CAD build for the part. Positions are in the model's coordinates, mm. A direction names the side the tool comes from. Coordinates: 2 decimals unless noted, no trailing zeros. Order: outer loops, then holes, each group sorted by start corner. A loop starts at its lowest first (then second) coordinate and runs counter-clockwise, first axis right, second up. Notation, with made-up numbers: M 87.25,64 L 140.25,64 A12 cw 140.25,73 Z; hole C 57.25,-2 d8. An arc over 180 degrees is marked long. Write item = value, one per line. Start each with the question number.
```python
from build123d import *

# Parameters (mm, degrees)
F0_W     = 82
F0_H     = 20
F0_R     = 2.5
F0_R_2   = 3
F1_DEPTH = 10
F2_W     = 57
F2_H     = 2
F3_DEPTH = 10


# Not quite as in the source:
# - a feature names something its author has since deleted; it is built from what else it names


with BuildPart() as f1:
    # F0 (on Top) → F1 (new body)
    with BuildSketch(Plane.XY):
        Rectangle(F0_W, F0_H)
        with Locations((26, -5)):
            Circle(F0_R, mode=Mode.SUBTRACT)
        with Locations((36, -5)):
            Circle(F0_R, mode=Mode.SUBTRACT)
        with Locations((-8, 0)):
            Circle(F0_R_2, mode=Mode.SUBTRACT)
    extrude(amount=F1_DEPTH)

    # F2 (on face) → F3 (cut)
    with BuildSketch(Plane.XY.offset(10)):
        Polygon((-16, 10), (-41, 10), (-41, -2), (-16, -2), (-16, 8), align=None)
        with Locations((12.5, 9)):
            Rectangle(F2_W, F2_H)
    extrude(amount=-F3_DEPTH, mode=Mode.SUBTRACT)


solid = f1.part
```
1. Slice it at D-D (y = -5). Write the cut outline in (x, z).
2. Slice it at A-A (y = 0). Write the cut outline in (x, z).
3. Slice it at B-B (x = -8). Write the cut outline in (y, z), plus the area to 3 significant figures.
4. Slice it at C-C (z = 2.5). Write the cut outline in (x, y).
5. Probe L1, parallel to Y at x = -8, z = 7.75; L2, parallel to Y at x = 36, z = 4.5; L3, parallel to X at y = -4, z = 0.75. List the from-to ranges inside material, lowest first.
6. 3-axis set-ups, long thin cutter, end or side, ignore diameter. For faces 1 (the flat face through (-41, -6, 5)), 2 (the flat face through (-16, 3, 5)): which of +Z, -Z, +X, -X, +Y, -Y reach the whole face in a straight line?
7. Mould opens along Y. For faces 3 (the flat face through (-29, -2, 5)), 4 (the flat face through (-1, -1, 10)), 5 (the cylindrical face through (24.16, -3.31, 4.93)) say: released by +Y, released by -Y, zero draft, split by the parting line, or undercut.
8. Flat gauge pins, fed straight in: pin 1 (5 mm diameter, centred on x = -32.5, z = 4, fed in from +Y); pin 2 (3.5 mm diameter, centred on x = -8, y = 0, fed in from +Z); pin 3 (3 mm diameter, centred on y = 0.5, z = 4.5, fed in from -X). Where does each tip first touch, or does it go through?
Calculated:
q1.outline = M -41,0 L 23.5,0 L 23.5,10 L -41,10 Z; M 28.5,0 L 33.5,0 L 33.5,10 L 28.5,10 Z; M 38.5,0 L 41,0 L 41,10 L 38.5,10 Z
q2.outline = M -16,0 L -11,0 L -11,10 L -16,10 Z; M -5,0 L 41,0 L 41,10 L -5,10 Z
q3.outline = M -10,0 L -3,0 L -3,10 L -10,10 Z; M 3,0 L 8,0 L 8,10 L 3,10 Z
q3.area = 120 mm²
q4.outline = M -41,-10 L 41,-10 L 41,8 L -16,8 L -16,-2 L -41,-2 Z; hole C -8,0 d6; hole C 26,-5 d5; hole C 36,-5 d5
q5.L1 = -10 to -3, 3 to 8
q5.L2 = -10 to -7.5, -2.5 to 8
q5.L3 = -41 to 23.71, 28.29 to 33.71, 38.29 to 41
q6.face_1 = +Z, -Z, -X, +Y, -Y
q6.face_2 = +Z, -Z, -X, +Y
q7.face_3 = released by +Y
q7.face_4 = zero draft
q7.face_5 = undercut
q8.pin_1 = -2
q8.pin_2 = through
q8.pin_3 = -16
